The model under review builds one solid part; all positions refer to its coordinate system, in mm. A direction names the side the tool comes from. Coordinates: 2 decimals unless noted, no trailing zeros. Write each loop counter-clockwise with the first axis right and the second up, starting at its lowest first coordinate (ties: lowest second). Pieces come first, ordered by that corner, then holes.
```python
from build123d import *

# Parameters (mm, degrees)
SKETCH1_R           = 15
BOSS_EXTRUDE1_DEPTH = 80
CUT_EXTRUDE2_START  = -60
CUT_EXTRUDE2_DEPTH  = 60


with BuildPart() as part:
    # Sketch1 → Boss-Extrude1 (new body)
    with BuildSketch(Plane(origin=(0, 0, 0), x_dir=(0, 0, -1), z_dir=(1, 0, 0))):
        Circle(SKETCH1_R)
    extrude(amount=BOSS_EXTRUDE1_DEPTH)

    # Sketch2 → Cut-Extrude2 (cut)
    with BuildSketch(Plane(origin=(80, 0, 0), x_dir=(0, 0, -1), z_dir=(1, 0, 0)).offset(CUT_EXTRUDE2_START)):
        with BuildLine():
            ThreePointArc((5, 14.142135624), (2.536529681, 14.783978395), (0, 15))
            ThreePointArc((0, 15), (-2.536529681, 14.783978395), (-5, 14.142135624))
            Line((-5, 14.142135624), (-5, 11))
            Line((-5, 11), (0, 11))
            Line((0, 11), (5, 11))
            Line((5, 11), (5, 14.142135624))
        make_face()
    extrude(amount=CUT_EXTRUDE2_DEPTH, mode=Mode.SUBTRACT)


solid = part.part
```
Item 1: For pin 1 (1.2 mm diameter, centred on y = 13, z = 0.5, fed in from +X); pin 2 (1 mm diameter, centred on x = 11.5, y = -2, fed in from +Z); pin 3 (1.5 mm diameter, centred on x = 11.5, z = 11.5, fed in from -Y), all flat-tipped, find the tip position at first contact; note any pin that passes through.
Solved:
pin 1: stops at x = 20
pin 2: stops at z = 14.92
pin 3: stops at y = -10.46
Item 2: Machinability: for faces 1 (the face through (0, 0, 0)), 2 (the face through (50, 13, -5)), which of the approach directions +Z, -Z, +X, -X, +Y, -Y give a long, thin tool a straight path to every point of the face, cutting with its end or side? Answer none if there is none.
Solved:
face 1: +Z, -Z, -X, +Y, -Y
face 2: +X, +Y
Item 3: Take a section at C-C, the plane y = -10.75. Write out the cut boundary in (x, z), plus the area to 3 significant figures.
Solved:
outline: (0, -10.46) - (80, -10.46) - (80, 10.46) - (0, 10.46) - close
area: 1,670 mm2
Item 4: Take a section at B-B, the plane x = 74.5. Write out the cut boundary in (y, z).
Solved:
outline: (11, -5) - (11, 5) - (14.14, 5) arc R15 ccw (long way) to (14.14, -5) - close
Item 5: Mouldability with a two-part tool opening along Z and no side actions: class faces 3 (the face through (80, 0, 0)), 4 (the face through (39.44, -14.643, 3.252)), 5 (the face through (50, 13, 5)) as pulls with the +Z half, pulls with the -Z half, needs draft (parallel to the pull), parting line crosses it, or undercut.
Solved:
face 3: needs draft
face 4: parting line crosses it
face 5: undercut
Item 6: Take a section at D-D, the plane z = -3.25. Write out the cut boundary in (x, y).
Solved:
outline: (0, -14.64) - (80, -14.64) - (80, 11) - (20, 11) - (20, 14.64) - (0, 14.64) - close
Item 7: Take a section at A-A, the plane z = 0. Write out the cut boundary in (x, y), plus the area to 3 significant figures.
Solved:
outline: (0, -15) - (80, -15) - (80, 11) - (20, 11) - (20, 15) - (0, 15) - close
area: 2,160 mm2
Item 8: To check wall thickness, follow line 1 along Z through (x, y) = (66, 0.5); line 2 along Y through (x, z) = (42, 0); line 3 along Z through (x, y) = (70, 12.5). State the ranges of each line that lie inside material, in increasing order.
Solved:
line 1: z = -14.99 to 14.99
line 2: y = -15 to 11
line 3: z = -8.29 to -5, 5 to 8.29
